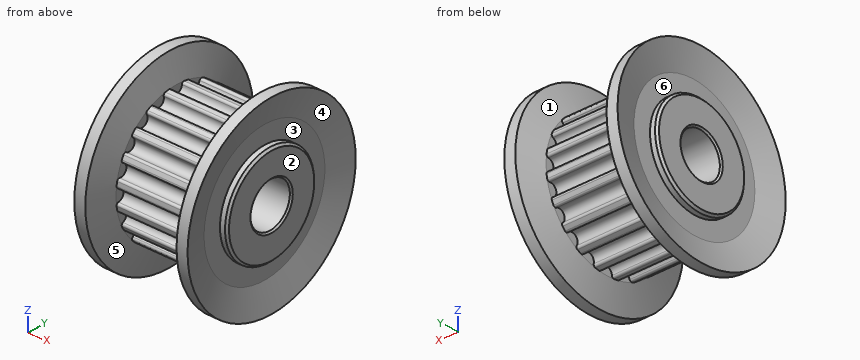
```python
from build123d import *

# Parameters (mm, degrees)
CUT_EXTRUDE_START        = 8.65
CUT_EXTRUDE_1_DEPTH      = 7
PATTERN_CIRCULAR_1_COUNT = 20
SKETCH_6_R               = 2
CUT_EXTRUDE_2_DEPTH      = 16.830034744
CHAMFER_1_SIZE           = 0.14


with BuildPart() as part:
    # 草图3 → 旋转1 (revolve)
    with BuildSketch(Plane.XY):
        Polygon((0, 0), (0, 4.31), (0.19, 4.5), (1.65, 4.5), (1.65, 6.11), (8.65, 6.11), (8.65, 4.5), (10.11, 4.5), (10.3, 4.31), (10.3, 0), align=None)
    revolve(axis=Axis((10.3, 0, 0), (-1, 0, 0)))

    # 草图4 → 切除-拉伸1 (cut)
    with BuildSketch(Plane(origin=(0, 0, 0), x_dir=(0, 0, -1), z_dir=(1, 0, 0)).offset(CUT_EXTRUDE_START)):
        with BuildLine():
            ThreePointArc((0.773818245, 6.060800716), (0, 6.11), (-0.773818245, 6.060800716))
            ThreePointArc((-0.773818245, 6.060800716), (-0.621157102, 6.016640443), (-0.548891698, 5.875101523))
            ThreePointArc((-0.548891698, 5.875101523), (0, 5.36), (0.548891698, 5.875101523))
            ThreePointArc((0.548891698, 5.875101523), (0.621157102, 6.016640443), (0.773818245, 6.060800716))
        make_face()
    cut_extrude_1 = extrude(amount=-CUT_EXTRUDE_1_DEPTH, mode=Mode.SUBTRACT)

    # 阵列(圆周)1: 切除-拉伸1 ×20 about axis
    pattern_circular_1_axis = Axis((0, 0, 0), (1, 0, 0))
    for i in range(1, PATTERN_CIRCULAR_1_COUNT):
        add(cut_extrude_1.rotate(pattern_circular_1_axis, i * 360 / PATTERN_CIRCULAR_1_COUNT), mode=Mode.SUBTRACT)

    # 草图5 → 旋转2 (revolve)
    with BuildSketch(Plane.XY, mode=Mode.PRIVATE) as revolve_2_sk:
        Polygon((1, 8.5), (1.65, 6.11), (1.65, 4.5), (0.65, 4.5), (0.65, 6.11), (0, 8.5), align=None)
        Polygon((9.65, 4.5), (8.65, 4.5), (8.65, 6.11), (9.3, 8.5), (10.3, 8.5), (9.65, 6.11), align=None)
    revolve(revolve_2_sk.sketch.rotate(Axis((0, 0, 0), (1, 0, 0)), 180), axis=Axis((0, 0, 0), (1, 0, 0)))

    # 草图6 → 切除-拉伸2 (cut, through all)
    with BuildSketch(Plane(origin=(0, 0, 0), x_dir=(0, 0, -1), z_dir=(1, 0, 0))):
        Circle(SKETCH_6_R)
    extrude(amount=CUT_EXTRUDE_2_DEPTH, mode=Mode.SUBTRACT)

    # 倒角1
    chamfer_1_edges = [part.edges().sort_by_distance(p)[0] for p in [
        (0, 0, 2),
        (10.3, 0, 2),
    ]]
    chamfer(chamfer_1_edges, length=CHAMFER_1_SIZE)


solid = part.part
```
Could you check a few things on this model? Use its own coordinates, in mm. Face numbers are marked on the shaded views. A direction names the side the tool comes from. Coordinates: 2 decimals unless noted, no trailing zeros. One line per question, with ' | ' between items. Start each with the question number.
1. Thinking about a two-plate mould opening in Y: for the marked faces 1, 2 and 3, which applies, pulls with the +Y half, pulls with the -Y half, needs draft (parallel to the pull), parting line crosses it, or undercut?
2. Please list where these lines run through material, in increasing order: line 1 along Z through (x, y) = (5.5, 0); line 2 along X through (y, z) = (-5, 1.25).
3. Will these pins go through, and if not, where does the flat tip stop? P1, Ø0.9, axis at y = 4, z = -5, coming from the +X side; P2, Ø0.9, axis at y = 4.5, z = -4, coming from the -X side; P3, Ø1.2, axis at y = -3.5, z = 4.5, coming from the +X side.
4. For the marked faces 4, 5 and 6, which set-ups out of +Z, -Z, +X, -X, +Y, -Y let a thin tool reach every point of the face, with its end or its side?
Return value:
1) face 1: parting line crosses it | face 2: needs draft | face 3: undercut
2) line 1: z = -5.36 to -2, 2 to 5.36 | line 2: x = 0.65 to 9.65
3) P1: stops at x = 9.85 | P2: stops at x = 0.55 | P3: stops at x = 9.7
4) face 4: +X | face 5: none | face 6: -X
